Can you work these out from the model? Positions are in its coordinate system, mm. Face numbers are marked on the shaded views. A direction names the side the tool comes from. Give positions to 0.01 mm unless a question says otherwise; leave off trailing zeros. Order: outer loops, then holes, each group sorted by start corner. A loop starts at its lowest first (then second) coordinate and runs counter-clockwise, first axis right, second up. Notation, with made-up numbers: (5.5, 87) - (64.5, 87) arc R17 ccw to (64.5, 116) - close; hole circle Ø5 at (-19, 63.5). An arc over 180 degrees is marked (long way). Use one line per item in the form item = value. Start each with the question number.
1) Suppose I cut it at A-A, the plane y = -11.5. Write out the boundary of the cut face in (x, z).
2) Please list where these lines run through material, in increasing order: probe 1 along Z at (x, y) = (-60.5, -22); probe 2 along X at (y, z) = (10, -11); probe 3 along Z at (x, y) = (-57.25, 15.5).
3) Which directions (+Z, -Z, +X, -X, +Y, -Y) give clear straight access to the entire face, cutting with the end or side of a thin tool? Please do the marked faces 5, 6 and 7.
4) Suppose I cut it at B-B, the plane x = -52. Write out the boundary of the cut face in (y, z), and give its area (3 significant figures).
5) For pin 1 (3 mm diameter, centred on x = -45.5, z = -14.5, fed in from +Y); pin 2 (3.5 mm diameter, centred on x = -45.01, y = 21.79, fed in from -Z); pin 3 (4 mm diameter, centred on x = -50.67, y = -14.86, fed in from -Z); pin 4 (10 mm diameter, centred on x = -59, z = -21, fed in from +Y), each with a flat end and sliding along its axis, tell me the tip position at first contact or that it passes through.
6) We'd pull the mould along Z, two halves only. Please class the marked faces 1, 2, 3 and 4: released by +Z, released by -Z, zero draft, split by the parting line, or undercut.
7) Suppose I cut it at C-C, the plane z = -21.5. Write out the boundary of the cut face in (x, y).
8) Suppose I cut it at D-D, the plane x = -42. Write out the boundary of the cut face in (y, z).
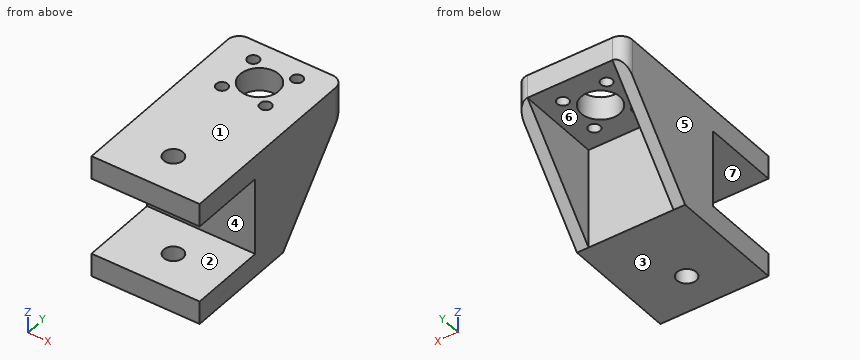
```python
from build123d import *

# Parameters (mm, degrees)
F0_W          = 22
F0_H          = 22
F0_R          = 1.5
F0_R_2        = 5
F1_DEPTH      = 6
F2_W          = 22
F2_H          = 32
F3_DEPTH      = 10
F4_W          = 22
F4_H          = 6
F5_DEPTH      = 20
F6_R          = 2.5
F7_DEPTH      = 32.001
F9_DEPTH      = 3
F11_DEPTH     = 3
F12_T1_DEPTH  = 21
F12_T6_DEPTH  = 5.7473088859
F12_S7_R      = 3
F12_T8_DEPTH  = 5
F12_T12_DEPTH = 5.7473088859
F12_S13_R     = 3
F12_T14_DEPTH = 5


# Not quite as in the source:
# - a fillet or chamfer that OpenCascade refuses, or shapes differently, is made with other operations: its cross-section is extruded or revolved along the edge and cut away or added
# - a feature of the source that left no trace in its solid (it failed there, or was rolled back) is left out


with BuildPart() as f1:
    # F0 (on Top) → F1 (new body)
    with BuildSketch(Plane.XY):
        with Locations((-50.6666042507, 16.1375404)):
            Rectangle(F0_W, F0_H)
        with Locations((-56.3234585002, 10.4806861505)):
            Circle(F0_R, mode=Mode.SUBTRACT)
        with Locations((-45.0097500012, 10.4806861505)):
            Circle(F0_R, mode=Mode.SUBTRACT)
        with Locations((-50.6666042507, 16.1375404)):
            Circle(F0_R_2, mode=Mode.SUBTRACT)
        with Locations((-56.3234585002, 21.7943946495)):
            Circle(F0_R, mode=Mode.SUBTRACT)
        with Locations((-45.0097500012, 21.7943946495)):
            Circle(F0_R, mode=Mode.SUBTRACT)
    extrude(amount=F1_DEPTH)

    # F2 (on face) → F3 (join)
    with BuildSketch(Plane.XZ.offset(-5.1375404)):
        with Locations((-50.6666042507, -10)):
            Rectangle(F2_W, F2_H)
    extrude(amount=F3_DEPTH)

    # F4 (on face) → F5 (join)
    with BuildSketch(Plane.XZ.offset(4.8624596)):
        with Locations((-50.6666042507, 3)):
            Rectangle(F4_W, F4_H)
        with Locations((-50.6666042507, -23)):
            Rectangle(F4_W, F4_H)
    extrude(amount=F5_DEPTH)

    # F6 (on face) → F7 (cut, through all)
    with BuildSketch(Plane.XY.offset(6)):
        with Locations((-50.6666042507, -14.8624596)):
            Circle(F6_R)
    extrude(amount=-F7_DEPTH, mode=Mode.SUBTRACT)

    # F8 (on face) → F9 (join)
    with BuildSketch(Plane(origin=(-61.6666042507, 0, 0), x_dir=(0, -1, 0), z_dir=(-1, 0, 0))):
        Polygon((-27.1375404, 0), (-5.1375404, -26), (-5.1375404, 0), align=None)
        Polygon((-5.1375404, 0), (-5.1375404, -26), (24.8624596, -26), (24.8624596, -20), (4.8624596, -20), (4.8624596, 0), (24.8624596, 0), (24.8624596, 6), (-27.1375404, 6), (-27.1375404, 0), align=None)
    extrude(amount=F9_DEPTH)

    # F10 (on face) → F11 (join)
    with BuildSketch(Plane.YZ.offset(-39.6666042507)):
        Polygon((5.1375404, 0), (5.1375404, -26), (27.1375404, 0), align=None)
        Polygon((-24.8624596, -26), (5.1375404, -26), (5.1375404, 0), (27.1375404, 0), (27.1375404, 6), (-24.8624596, 6), (-24.8624596, 0), (-4.8624596, 0), (-4.8624596, -20), (-24.8624596, -20), align=None)
    extrude(amount=F11_DEPTH)

    # F12: fillet of radius 3 on 4 edges, made by hand

    # F12_s2 → F12_t1 (cut)
    with BuildSketch(Plane.XY.offset(-7.5)):
        with BuildLine():
            ThreePointArc((-61.6666042507, 27.1375404), (-63.7879245942, 26.2588607436), (-64.6666042507, 24.1375404))
            Line((-64.6666042507, 24.1375404), (-64.6666042507, 27.1375404))
            Line((-64.6666042507, 27.1375404), (-61.6666042507, 27.1375404))
        make_face()
        with BuildLine():
            ThreePointArc((-39.6666042507, 27.1375404), (-37.5452839071, 26.2588607436), (-36.6666042507, 24.1375404))
            Line((-36.6666042507, 24.1375404), (-36.6666042507, 27.1375404))
            Line((-36.6666042507, 27.1375404), (-39.6666042507, 27.1375404))
        make_face()
    extrude(amount=F12_T1_DEPTH, mode=Mode.SUBTRACT)


with BuildPart() as f12_tool4:
    # F12_s5 → F12_t6 (new body)
    with BuildSketch(Plane.YZ.offset(-61.6666042507)):
        with BuildLine():
            ThreePointArc((27.1375404, 1.0989235543), (26.9544958992, 0.0670506378), (26.4276992561, -0.8389031701))
            Line((26.4276992561, -0.8389031701), (27.1375404, 0))
            Line((27.1375404, 0), (27.1375404, 1.0989235543))
        make_face()
    extrude(amount=-F12_T6_DEPTH)

    # F12_s7 → F12_t8 (cut, symmetric)
    with BuildSketch(Plane.XY.offset(0.1)):
        with Locations((-61.6666042507, 24.1375404)):
            Circle(F12_S7_R)
    extrude(amount=F12_T8_DEPTH, both=True, mode=Mode.SUBTRACT)


with BuildPart() as f1_1:
    add(f1.part)

    # F12_t3: cut F12_tool4
    add(f12_tool4.part, mode=Mode.SUBTRACT)


with BuildPart() as f12_tool10:
    # F12_s11 → F12_t12 (new body)
    with BuildSketch(Plane.YZ.offset(-39.6666042507)):
        with BuildLine():
            ThreePointArc((27.1375404, 1.0989235543), (26.9544958992, 0.0670506378), (26.4276992561, -0.8389031701))
            Line((26.4276992561, -0.8389031701), (27.1375404, 0))
            Line((27.1375404, 0), (27.1375404, 1.0989235543))
        make_face()
    extrude(amount=F12_T12_DEPTH)

    # F12_s13 → F12_t14 (cut, symmetric)
    with BuildSketch(Plane.XY.offset(0.1)):
        with Locations((-39.6666042507, 24.1375404)):
            Circle(F12_S13_R)
    extrude(amount=F12_T14_DEPTH, both=True, mode=Mode.SUBTRACT)


with BuildPart() as f1_2:
    add(f1_1.part)

    # F12_t9: cut F12_tool10
    add(f12_tool10.part, mode=Mode.SUBTRACT)


solid = f1_2.part
```
Result sheet:
q1.outline = (-64.67, -26) - (-36.67, -26) - (-36.67, -20) - (-64.67, -20) - close; (-64.67, 0) - (-36.67, 0) - (-36.67, 6) - (-64.67, 6) - close
q2.probe_1 = -26 to -20, 0 to 6
q2.probe_2 = -64.67 to -61.67, -39.67 to -36.67
q2.probe_3 = 0 to 6
q3.face_5 = +Z, -Z, -X, +Y, -Y
q3.face_6 = -Z, +Y
q3.face_7 = +X, -X, -Y
q4.outline = (-24.86, -26) - (-16.98, -26) - (-16.98, -20) - (-24.86, -20) - close; (-24.86, 0) - (-16.98, 0) - (-16.98, 6) - (-24.86, 6) - close; (-12.75, -26) - (5.14, -26) - (5.14, 0) - (11.32, 0) - (11.32, 6) - (-12.75, 6) - (-12.75, 0) - (-4.86, 0) - (-4.86, -20) - (-12.75, -20) - close; (20.96, 0) - (27.14, 0) - (27.14, 6) - (20.96, 6) - close
q4.area = 583 mm²
q5.pin_1 = 5.14
q5.pin_2 = 0
q5.pin_3 = through
q5.pin_4 = 12.95
q6.face_1 = released by +Z
q6.face_2 = undercut
q6.face_3 = released by -Z
q6.face_4 = undercut
q7.outline = (-64.67, -24.86) - (-36.67, -24.86) - (-36.67, 8.95) - (-39.67, 8.95) - (-39.67, 5.14) - (-61.67, 5.14) - (-61.67, 8.95) - (-64.67, 8.95) - close; hole circle Ø5 at (-50.67, -14.86)
q8.outline = (-24.86, -26) - (5.14, -26) - (5.14, 0) - (27.14, 0) - (27.14, 6) - (-24.86, 6) - (-24.86, 0) - (-4.86, 0) - (-4.86, -20) - (-24.86, -20) - close
